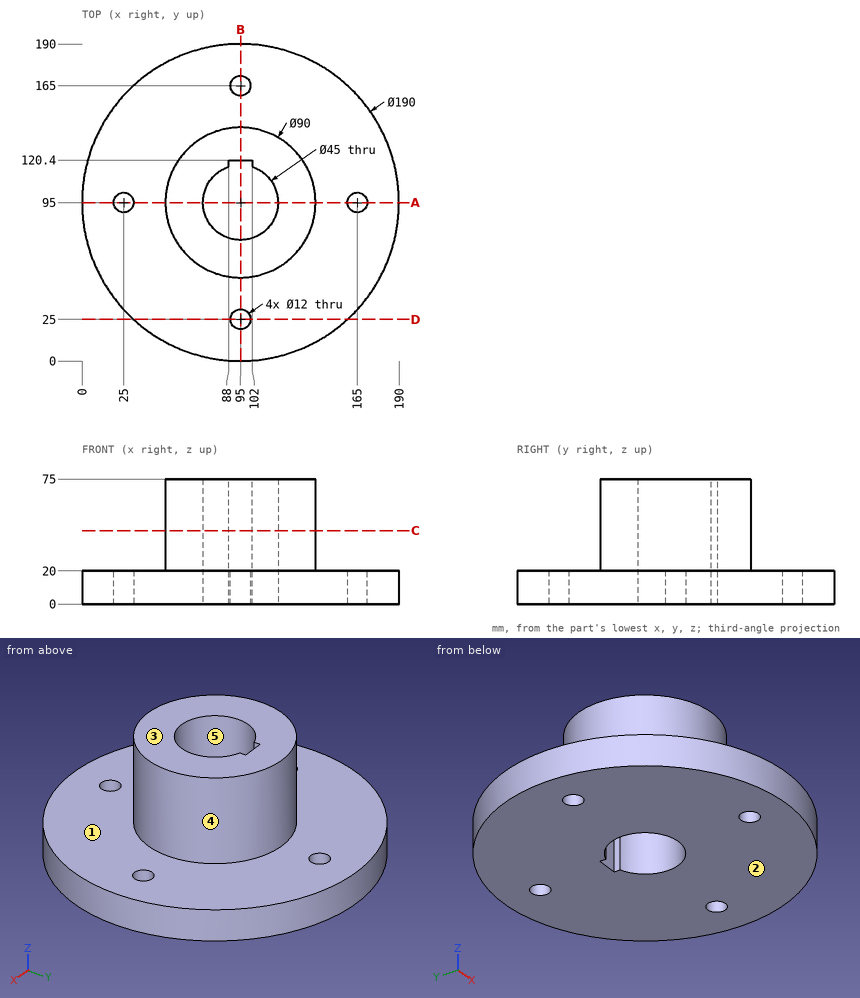
Input: dimensioned drawing with shaded views. Units: mm. Origin: part minimum x, y, z. A direction names the side the tool comes from. Round coordinates to 2 decimals unless told otherwise and drop trailing zeros. Loops run counter-clockwise (first coordinate to the right, second up) from the corner with the lowest first, then second, coordinate; pieces in that order, holes last. Notation, with made-up numbers: (18.25, 83) -> (22.25, 83) arc R18 ccw to (22.25, 91) -> close; hole circle Ø1 at (-1.5, 34.25). An arc over 180 degrees is marked (long way). Answer as a JSON object with one key per item and string values. Group by question number.
Q1. Section query A-A (y = 95). Output: boundary loops of the cut face in (x, z), plus the area to 4 significant figures.
Q2. Section query C-C (z = 44). Output: boundary loops of the cut face in (x, y).
Q3. Section query B-B (x = 95). Output: boundary loops of the cut face in (y, z).
Q4. Section query D-D (y = 25). Output: boundary loops of the cut face in (x, z), plus the area to 3 significant figures.
Q5. Ray query, line 1 (Y direction, x = 95, z = 9.5); line 2 (Z direction, x = 117, y = 40); line 3 (X direction, y = 25, z = 6). Return the intervals inside material, ascending. Write a range as from..to.
Q6. Mould query, pull axis X, two halves, no side actions, for the marked faces 3, 4 and 5. Classes: pulls with the +X half, pulls with the -X half, needs draft (parallel to the pull), parting line crosses it, or undercut.
Q7. Contact query for flat-ended pins moving along their axis: P1, Ø8, axis at x = 41, y = 140, coming from the +Z side; P2, Ø9.5, axis at x = 95, y = 25, coming from the +Z side; P3, Ø12, axis at x = 113.5, z = 66.5, coming from the -Y side; P4, Ø4.5, axis at y = 118.5, z = 43, coming from the +X side. Output: stop coordinate, or through.
Q8. Access query for the marked faces 1 and 2. Directions: +Z, -Z, +X, -X, +Y, -Y. A direction counts if a zero-diameter tool reaches every point of the face in a straight line with its end or side. Return the directions, or none.
Completed:
{
 "1": {"outline": "(0, 0) -> (19, 0) -> (19, 20) -> (0, 20) -> close; (31, 0) -> (72.5, 0) -> (72.5, 75) -> (50, 75) -> (50, 20) -> (31, 20) -> close; (117.5, 0) -> (159, 0) -> (159, 20) -> (140, 20) -> (140, 75) -> (117.5, 75) -> close; (171, 0) -> (190, 0) -> (190, 20) -> (171, 20) -> close", "area": "4,895 mm²"},
 "2": {"outline": "circle Ø90 at (95, 95); hole (88, 116.38) arc R22.5 ccw (long way) to (102, 116.38) -> (102, 120.4) -> (88, 120.4) -> close"},
 "3": {"outline": "(0, 0) -> (19, 0) -> (19, 20) -> (0, 20) -> close; (31, 0) -> (72.5, 0) -> (72.5, 75) -> (50, 75) -> (50, 20) -> (31, 20) -> close; (120.4, 0) -> (159, 0) -> (159, 20) -> (140, 20) -> (140, 75) -> (120.4, 75) -> close; (171, 0) -> (190, 0) -> (190, 20) -> (171, 20) -> close"},
 "4": {"outline": "(30.77, 0) -> (89, 0) -> (89, 20) -> (30.77, 20) -> close; (101, 0) -> (159.23, 0) -> (159.23, 20) -> (101, 20) -> close", "area": "2,330 mm²"},
 "5": {"line 1": "0..19, 31..72.5, 120.4..159, 171..190", "line 2": "0..20", "line 3": "30.77..89, 101..159.23"},
 "6": {"face 3": "needs draft", "face 4": "parting line crosses it", "face 5": "undercut"},
 "7": {"P1": "z = 20", "P2": "through", "P3": "y = 51.77", "P4": "x = 134.67"},
 "8": {"face 1": "+Z", "face 2": "-Z, +X, -X, +Y, -Y"}
}
